Verification items for the finished model (mm, model axes). A direction names the side the tool comes from. Round coordinates to 2 decimals unless told otherwise and drop trailing zeros. Write each loop counter-clockwise with the first axis right and the second up, starting at its lowest first coordinate (ties: lowest second). Pieces come first, ordered by that corner, then holes. Notation, with made-up numbers: (-37.75, 82.5) - (-29.75, 82.5) arc R35 cw to (-29.75, 116.5) - close; hole circle Ø1 at (-4.75, 70). An arc over 180 degrees is marked (long way). Answer as a JSON object with one key per item and string values.
```python
from build123d import *

# Parameters (mm, degrees)
SKETCH1_W           = 40
SKETCH1_H           = 40
BOSS_EXTRUDE1_DEPTH = 3
SKETCH2_R           = 0.5


with BuildPart() as part:
    # Sketch1 → Boss-Extrude1 (new body)
    with BuildSketch(Plane(origin=(0, 0, 0), x_dir=(1, 0, 0), z_dir=(0, 1, 0))):
        Rectangle(SKETCH1_W, SKETCH1_H)
    extrude(amount=BOSS_EXTRUDE1_DEPTH)

    # Sweep1: sweep along a path in Sketch3
    with BuildLine(Plane.XY.offset(18.5)) as sweep1_path:
        Line((20, 1.5), (20.711014952, 1.5))
        ThreePointArc((20.711014952, 1.5), (24.225698973, 2.955829789), (25.681528762, 6.47051381))
    # Sketch2 → Sweep1 (sweep)
    with BuildSketch(Plane(origin=(20, 0, 0), x_dir=(0, 0, -1), z_dir=(1, 0, 0))):
        with Locations((-18.5, 1.5)):
            Circle(SKETCH2_R)
    sweep1 = sweep(path=sweep1_path.line)

    # Mirror1: Sweep1 across plane
    add(sweep1.mirror(Plane.XY))


solid = part.part
```
1. Go/stop test with flat-tipped pins: pin 1 (3 mm diameter, centred on x = -8.5, z = -7, fed in from +Y); pin 2 (2.5 mm diameter, centred on y = 1, z = 0, fed in from +X). Record where each tip stops, or that it passes through.
Completed:
{"pin 1": "stops at y = 3", "pin 2": "stops at x = 20"}
2. Mould release check, pull along Z, two halves, no side actions. Record for faces 1 (the face through (0, 1, -20)), 2 (the face through (20, 1, 0)), 3 (the face through (25.7, 6.471, 18.5)): released by +Z, released by -Z, zero draft, split by the parting line, or undercut.
Completed:
{"face 1": "released by -Z", "face 2": "undercut", "face 3": "zero draft"}
3. Material ranges on probe 1 along Y at (x, z) = (-17.5, -17); probe 2 along X at (y, z) = (1.25, 0.5), recorded low to high. Write a range as from..to.
Completed:
{"probe 1": "y = 0..3", "probe 2": "x = -20..20"}
4. Cross-section at B-B (x = -4.5). Record the boundary of the cut face in (y, z).
Completed:
{"outline": "(0, -20) - (3, -20) - (3, 20) - (0, 20) - close"}
5. Cross-section at C-C (z = 0.5). Record the boundary of the cut face in (x, y).
Completed:
{"outline": "(-20, 0) - (20, 0) - (20, 3) - (-20, 3) - close"}
6. Cross-section at A-A (z = 18.5). Record the boundary of the cut face in (x, y), plus the area to 3 significant figures.
Completed:
{"outline": "(-20, 0) - (20, 0) - (20, 1) - (20.71, 1) arc R5.47 ccw to (26.18, 6.47) - (25.18, 6.47) arc R4.47 cw to (20.71, 2) - (20, 2) - (20, 3) - (-20, 3) - close", "area": "129 mm^2"}
7. Access from +Z, -Z, +X, -X, +Y, -Y to the whole of each face (thin tool, end or side, straight path). Record for faces 4 (the face through (0, 1, 20)), 5 (the face through (20.36, 1.65, 18.023)).
Completed:
{"face 4": "+Z, +X, -X, +Y, -Y", "face 5": "none"}
